CAD build for the part. Positions are in the model's coordinates, mm. Round coordinates to 2 decimals unless told otherwise and drop trailing zeros. Write each loop counter-clockwise with the first axis right and the second up, starting at its lowest first coordinate (ties: lowest second). Pieces come first, ordered by that corner, then holes. Notation, with made-up numbers: (26, -26.5) -> (75, -26.5) arc R12 cw to (75, -21.5) -> close; hole circle Ø3 at (40, -18). An arc over 180 degrees is marked (long way). Put each result on its own line as item: value. Start each with the question number.
1. Drill centre lines: line 1 (Z direction, x = -15, y = -30); line 2 (Z direction, x = 22.5, y = -57.5); line 3 (Y direction, x = 4, z = -76). Where is each one in solid material? Low to high. Write a range as from..to.
2. Flat gauge pins, fed straight in: P1, Ø2, axis at y = -21, z = 1370.5, coming from the +X side; P2, Ø4, axis at y = 25.5, z = -47.5, coming from the -X side; P3, Ø12, axis at x = 5.5, y = -49.5, coming from the -Z side. Where does each tip first touch, or does it go through?
3. Saw through at B-B on x = 0. List the corners of the cut face in (y, z).
4. Saw through at D-D on z = 369. List the corners of the cut face in (x, y).
5. Saw through at A-A on y = 0. List the corners of the cut face in (x, z).
6. Saw through at C-C on z = 1919. List the corners of the cut face in (x, y), and give its area (3 significant figures).
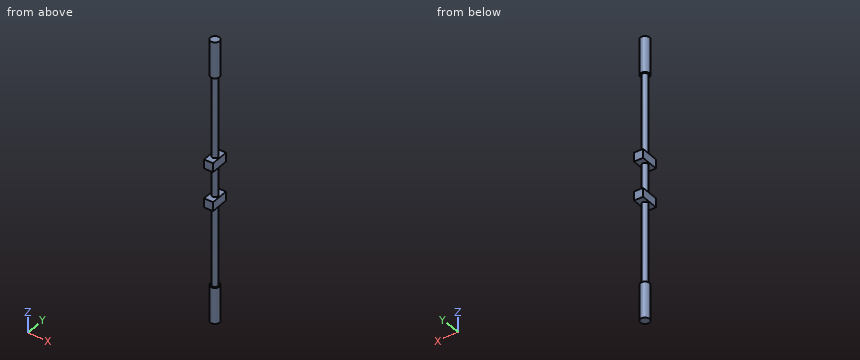
from build123d import *

# Parameters (mm, degrees)
SKETCH1_R           = 25.4
BOSS_EXTRUDE1_DEPTH = 1778
SKETCH2_R           = 38.1
BOSS_EXTRUDE2_DEPTH = 304.8
BOSS_EXTRUDE3_START = 304.8
SKETCH3_R           = 38.1
BOSS_EXTRUDE3_DEPTH = 304.8
SKETCH4_W           = 76.2
SKETCH4_H           = 76.2
BOSS_EXTRUDE4_DEPTH = 76.2


with BuildPart() as part:
    # Sketch1 → Boss-Extrude1 (new body)
    with BuildSketch(Plane.XY):
        Circle(SKETCH1_R)
    extrude(amount=BOSS_EXTRUDE1_DEPTH)

    # Sketch2 → Boss-Extrude2 (add)
    with BuildSketch(Plane.XY.offset(1778)):
        with Locations(Location((0, 0, 0), (0, 0, 180))):
            Circle(SKETCH2_R)
    extrude(amount=BOSS_EXTRUDE2_DEPTH)

    # Sketch3 → Boss-Extrude3 (add)
    with BuildSketch(Plane(origin=(0, 0, 0), x_dir=(-1, 0, 0), z_dir=(0, 0, -1)).offset(BOSS_EXTRUDE3_START)):
        Circle(SKETCH3_R)
    extrude(amount=-BOSS_EXTRUDE3_DEPTH)

    # Sketch4 → Boss-Extrude4 (add, symmetric)
    with BuildSketch(Plane(origin=(0, 0, 0), x_dir=(1, 0, 0), z_dir=(0, 1, 0))):
        with Locations((0, -1054.1)):
            Rectangle(SKETCH4_W, SKETCH4_H)
        with Locations((0, -723.9)):
            Rectangle(SKETCH4_W, SKETCH4_H)
    extrude(amount=BOSS_EXTRUDE4_DEPTH, both=True)


solid = part.part
Return value:
1. line 1: z = -304.8..0, 685.8..762, 1016..1092.2, 1778..2082.8
1. line 2: z = 685.8..762, 1016..1092.2
1. line 3: y = -37.89..37.89
2. P1: stops at x = 15.66
2. P2: stops at x = -29.99
2. P3: stops at z = 685.8
3. outline: (-76.2, 685.8) -> (-25.4, 685.8) -> (-25.4, 0) -> (-38.1, 0) -> (-38.1, -304.8) -> (38.1, -304.8) -> (38.1, 0) -> (25.4, 0) -> (25.4, 685.8) -> (76.2, 685.8) -> (76.2, 762) -> (25.4, 762) -> (25.4, 1016) -> (76.2, 1016) -> (76.2, 1092.2) -> (25.4, 1092.2) -> (25.4, 1778) -> (38.1, 1778) -> (38.1, 2082.8) -> (-38.1, 2082.8) -> (-38.1, 1778) -> (-25.4, 1778) -> (-25.4, 1092.2) -> (-76.2, 1092.2) -> (-76.2, 1016) -> (-25.4, 1016) -> (-25.4, 762) -> (-76.2, 762) -> close
4. outline: circle Ø50.8 at (0, 0)
5. outline: (-38.1, -304.8) -> (38.1, -304.8) -> (38.1, 0) -> (25.4, 0) -> (25.4, 685.8) -> (38.1, 685.8) -> (38.1, 762) -> (25.4, 762) -> (25.4, 1016) -> (38.1, 1016) -> (38.1, 1092.2) -> (25.4, 1092.2) -> (25.4, 1778) -> (38.1, 1778) -> (38.1, 2082.8) -> (-38.1, 2082.8) -> (-38.1, 1778) -> (-25.4, 1778) -> (-25.4, 1092.2) -> (-38.1, 1092.2) -> (-38.1, 1016) -> (-25.4, 1016) -> (-25.4, 762) -> (-38.1, 762) -> (-38.1, 685.8) -> (-25.4, 685.8) -> (-25.4, 0) -> (-38.1, 0) -> close
6. outline: circle Ø76.2 at (0, 0)
6. area: 4,560 mm^2
